from build123d import *

# Parameters (mm, degrees)
SKETCH_W        = 100
SKETCH_H        = 20
PAD_DEPTH       = 370
SKETCH001_W     = 100
SKETCH001_H     = 70
PAD001_DEPTH    = 10
SKETCH002_W     = 57
SKETCH002_H     = 57
PAD002_DEPTH    = 56
SKETCH003_W     = 15
SKETCH003_H     = 310
PAD003_DEPTH    = 15
SKETCH004_R     = 6
PAD004_DEPTH    = 370
SKETCH005_R     = 4
POCKET_DEPTH    = 15
POCKET001_DEPTH = 50
POCKET002_DEPTH = 310


with BuildPart() as part:
    # Sketch → Pad (new body)
    with BuildSketch(Plane.XZ):
        Rectangle(SKETCH_W, SKETCH_H)
    extrude(amount=PAD_DEPTH)

    # Sketch001 (on Face6 of Pad) → Pad001 (join)
    with BuildSketch(Plane.XZ.offset(370)):
        with Locations((0, 25)):
            Rectangle(SKETCH001_W, SKETCH001_H)
    extrude(amount=PAD001_DEPTH)

    # Sketch002 (on Face11 of Pad001) → Pad002 (join)
    with BuildSketch(Plane.XZ.offset(380)):
        with Locations((0, 28.5)):
            Rectangle(SKETCH002_W, SKETCH002_H)
    extrude(amount=PAD002_DEPTH)

    # Sketch003 (on Face1 of Pad002) → Pad003 (join)
    with BuildSketch(Plane(origin=(0, 0, 10), x_dir=(-1, 0, 0), z_dir=(0, 0, 1))):
        with Locations((-30, 175)):
            Rectangle(SKETCH003_W, SKETCH003_H)
        with Locations((30, 175)):
            Rectangle(SKETCH003_W, SKETCH003_H)
    extrude(amount=PAD003_DEPTH)

    # Sketch004 (on Face4 of Pad003) → Pad004 (join)
    with BuildSketch(Plane(origin=(0, -370, 0), x_dir=(1, 0, 0), z_dir=(0, 1, 0))):
        with Locations((0, -28.5)):
            Circle(SKETCH004_R)
    extrude(amount=PAD004_DEPTH)

    # Sketch005 (on Face14 of Pad004) → Pocket (cut)
    with BuildSketch(Plane(origin=(0, 0, -10), x_dir=(1, 0, 0), z_dir=(0, 0, -1))):
        with Locations((-25, 10)):
            Circle(SKETCH005_R)
        with Locations((25, 10)):
            Circle(SKETCH005_R)
        with Locations((25, 35)):
            Circle(SKETCH005_R)
        with Locations((-25, 35)):
            Circle(SKETCH005_R)
        with Locations((-25, 93)):
            Circle(SKETCH005_R)
        with Locations((-25, 68)):
            Circle(SKETCH005_R)
        with Locations((25, 93)):
            Circle(SKETCH005_R)
        with Locations((25, 68)):
            Circle(SKETCH005_R)
    extrude(amount=-POCKET_DEPTH, mode=Mode.SUBTRACT)

    # Sketch006 (on Face44 of Pocket) → Pocket001 (cut)
    with BuildSketch(Plane.XZ.offset(436)):
        with BuildLine():
            ThreePointArc((-28.5, 48), (-22.136039, 50.636039), (-19.5, 57))
            Line((-19.5, 57), (-28.5, 57))
            Line((-28.5, 57), (-28.5, 48))
        make_face()
        with BuildLine():
            ThreePointArc((19.5, 57), (22.136039, 50.636039), (28.5, 48))
            Line((28.5, 48), (28.5, 57))
            Line((28.5, 57), (19.5, 57))
        make_face()
        with BuildLine():
            ThreePointArc((28.5, 9), (22.136039, 6.363961), (19.5, 0))
            Line((28.5, 0), (19.5, 0))
            Line((28.5, 0), (28.5, 9))
        make_face()
        with BuildLine():
            ThreePointArc((-19.5, 0), (-22.136039, 6.363961), (-28.5, 9))
            Line((-28.5, 9), (-28.5, 0))
            Line((-19.5, 0), (-28.5, 0))
        make_face()
    extrude(amount=-POCKET001_DEPTH, mode=Mode.SUBTRACT)

    # Sketch007 (on Face7 of Pocket001) → Pocket002 (cut)
    with BuildSketch(Plane(origin=(0, -20, 0), x_dir=(1, 0, 0), z_dir=(0, 1, 0))):
        Polygon((-37.5, -22.5), (-35, -25), (-37.5, -25), align=None)
        Polygon((-37.5, -19.7), (-35, -17.2), (-35, -15.2), (-37.5, -12.7), align=None)
        Polygon((22.5, -22.5), (25, -25), (22.5, -25), align=None)
        Polygon((22.5, -19.7), (25, -17.2), (25, -15.2), (22.5, -12.7), align=None)
        Polygon((-22.5, -22.5), (-25, -25), (-22.5, -25), align=None)
        Polygon((-22.5, -19.7), (-25, -17.2), (-25, -15.2), (-22.5, -12.7), align=None)
        Polygon((37.5, -22.5), (35, -25), (37.5, -25), align=None)
        Polygon((37.5, -19.7), (35, -17.2), (35, -15.2), (37.5, -12.7), align=None)
    extrude(amount=-POCKET002_DEPTH, mode=Mode.SUBTRACT)


solid = part.part
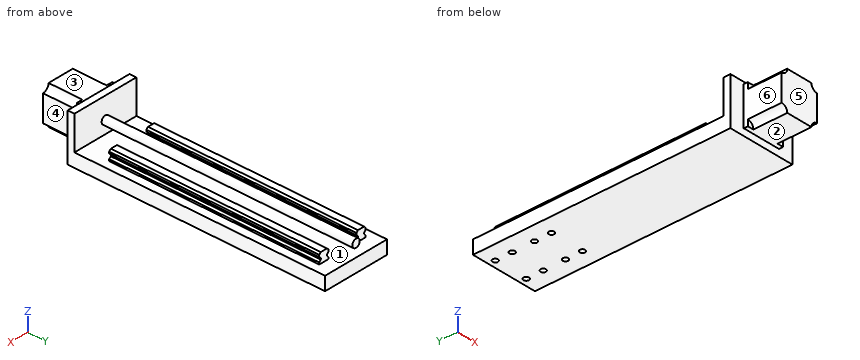
Work out the finished part from the listing and answer in its coordinate system (mm). Face numbers are marked on the shaded views. A direction names the side the tool comes from. Give positions to 0.01 mm unless a question says otherwise; leave off trailing zeros. Loops run counter-clockwise (first coordinate to the right, second up) from the corner with the lowest first, then second, coordinate; pieces in that order, holes last. Notation, with made-up numbers: M 52,72 L 66,72 A33 ccw 66,111 Z; hole C 1.25,22 d2. An arc over 180 degrees is marked long. Use CSV: the item, a comma, the result in double quotes.
1) Given P1, Ø2, axis at x = -21, z = 36.5, coming from the +Y side; P2, Ø1, axis at y = -126.5, z = 16, coming from the -X side; P3, Ø2.5, axis at x = 24, y = -11.5, coming from the -Z side, each flat-ended and moving along its own axis, determine where each tip first touches the part or whether it passes through.
Answer:
P1,"y = -370"
P2,"x = -35"
P3,"z = 5"
2) Consider L1, parallel to X at y = -10, z = -0.5; L2, parallel to Y at x = -25, z = 1; L3, parallel to Y at x = -25, z = -2. Determine where each line is inside the solid, lowest interval first.
Answer:
L1,"-50 to -29, -21 to 21, 29 to 50"
L2,"-386 to -97, -89 to -72, -64 to -39, -31 to -14, -6 to 0"
L3,"-380 to -97, -89 to -72, -64 to -39, -31 to -14, -6 to 0"
3) Which of the six approach directions +Z, -Z, +X, -X, +Y, -Y give full straight-line access (tool end or side, diameter ignored) to the marked faces 4, 5 and 6?
Answer:
face 4,"+Z, -Z, +X, -Y"
face 5,"+Z, -Z, +X, -X, -Y"
face 6,"+Z, -Z, -X, -Y"
4) Find section D-D on z = 39.5. Write down the section's boundary in (x, y).
Answer:
outline,"M -50,-380 L -28.5,-380 L -28.5,-436 L 28.5,-436 L 28.5,-380 L 50,-380 L 50,-370 L -50,-370 Z"
5) Find section B-B on z = -4.5. Give the number of separate pieces and of enclosed holes in the cut face, plus the area to 3 significant figures.
Answer:
separate pieces,"1"
enclosed holes,"8"
area,"37,600 mm^2"
6) Find section A-A on y = -10. Write down the section's boundary in (x, z), plus the area to 3 significant figures.
Answer:
outline,"M -50,-10 L -29,-10 L -29,5 L -21,5 L -21,-10 L 21,-10 L 21,5 L 29,5 L 29,-10 L 50,-10 L 50,10 L -50,10 Z; C 0,28.5 d12"
area,"1,870 mm^2"
7) Determine the mould class of the marked faces 1, 2 and 3 for opening direction Z: released by +Z, released by -Z, zero draft, split by the parting line, or undercut.
Answer:
face 1,"undercut"
face 2,"released by -Z"
face 3,"released by +Z"
8) Find section C-C on x = 0. Write down the section's boundary in (y, z).
Answer:
outline,"M -436,0 L -380,0 L -380,-10 L 0,-10 L 0,10 L -370,10 L -370,22.5 L 0,22.5 L 0,34.5 L -370,34.5 L -370,60 L -380,60 L -380,57 L -436,57 Z"
